from build123d import *

# Parameters (mm, degrees)
F1_DEPTH = 2
F0_R     = 1
F2_DEPTH = 1.2
F3_DEPTH = 5


with BuildPart() as f1:
    # F0 (on Front) → F1 (new body)
    with BuildSketch(Plane.XZ):
        with BuildLine():
            Line((-7.5, -4.5), (7.5, -4.5))
            ThreePointArc((7.5, -4.5), (8.914214, -3.914214), (9.5, -2.5))
            Line((9.5, -2.5), (9.5, 2.5))
            ThreePointArc((9.5, 2.5), (8.914214, 3.914214), (7.5, 4.5))
            Line((7.5, 4.5), (-7.5, 4.5))
            ThreePointArc((-7.5, 4.5), (-8.914214, 3.914214), (-9.5, 2.5))
            Line((-9.5, 2.5), (-9.5, -2.5))
            ThreePointArc((-9.5, -2.5), (-8.914214, -3.914214), (-7.5, -4.5))
        make_face()
        with BuildLine():
            ThreePointArc((8, -1), (7.414214, -2.414214), (6, -3))
            Line((6, -3), (-6, -3))
            ThreePointArc((-6, -3), (-7.414214, -2.414214), (-8, -1))
            Line((-8, -1), (-8, 1))
            ThreePointArc((-8, 1), (-7.414214, 2.414214), (-6, 3))
            Line((-6, 3), (6, 3))
            ThreePointArc((6, 3), (7.414214, 2.414214), (8, 1))
            Line((8, 1), (8, -1))
        make_face(mode=Mode.SUBTRACT)
    extrude(amount=F1_DEPTH)

    # F0 (on Front) → F2 (join)
    with BuildSketch(Plane.XZ):
        with BuildLine():
            Line((-6, -3), (6, -3))
            ThreePointArc((6, -3), (7.414214, -2.414214), (8, -1))
            Line((8, -1), (8, 1))
            ThreePointArc((8, 1), (7.414214, 2.414214), (6, 3))
            Line((6, 3), (-6, 3))
            ThreePointArc((-6, 3), (-7.414214, 2.414214), (-8, 1))
            Line((-8, 1), (-8, -1))
            ThreePointArc((-8, -1), (-7.414214, -2.414214), (-6, -3))
        make_face()
        Circle(F0_R, mode=Mode.SUBTRACT)
    extrude(amount=F2_DEPTH)

    # F0 (on Front) → F3 (join)
    with BuildSketch(Plane.XZ):
        Circle(F0_R)
    extrude(amount=F3_DEPTH)


solid = f1.part
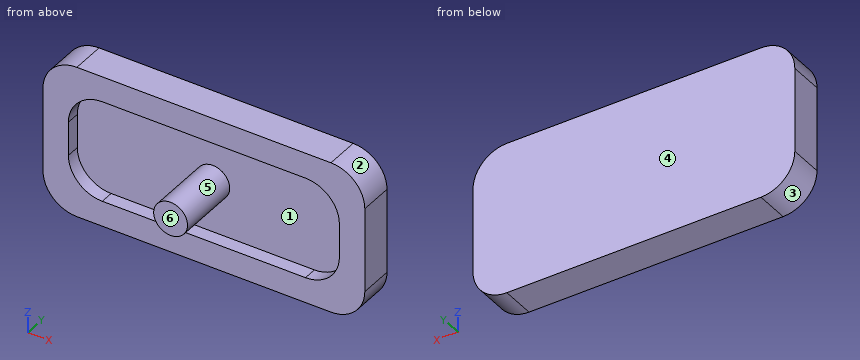
The listing builds one solid part. Answer for the finished solid, in the listing's coordinates (mm). Face numbers are marked on the shaded views. A direction names the side the tool comes from. Give positions to 0.01 mm unless a question says otherwise; leave off trailing zeros. Order: outer loops, then holes, each group sorted by start corner. A loop starts at its lowest first (then second) coordinate and runs counter-clockwise, first axis right, second up. Notation, with made-up numbers: (77.5, 20.5) - (83.5, 20.5) arc R14 ccw to (83.5, 33.5) - close; hole circle Ø7 at (-40, 56.5). An arc over 180 degrees is marked (long way). Use one line per item in the form item = value.
1) The mould has two halves that part along Z. Classify the marked faces 1, 2, 3 and 4: released by +Z, released by -Z, zero draft, split by the parting line, or undercut.
Verdict:
face_1 = undercut
face_2 = released by +Z
face_3 = released by -Z
face_4 = zero draft
2) For the marked faces 5 and 6, determine the directions among +Z, -Z, +X, -X, +Y, -Y from which every point of the face is accessible in a straight line to the end or side of a thin tool.
Verdict:
face_5 = -Y
face_6 = +Z, -Z, +X, -X, -Y
3) Find section B-B on z = 0. Determine the outline of the cut face in (x, y).
Verdict:
outline = (-9.5, -2) - (-8, -2) - (-8, -1.2) - (-1, -1.2) - (-1, -5) - (1, -5) - (1, -1.2) - (8, -1.2) - (8, -2) - (9.5, -2) - (9.5, 0) - (-9.5, 0) - close
4) Find section C-C on y = -4.6. Determine the outline of the cut face in (x, z).
Verdict:
outline = circle Ø2 at (0, 0)
5) Find section A-A on x = 0. Determine the outline of the cut face in (y, z), and give its area (3 significant figures).
Verdict:
outline = (-5, -1) - (-1.2, -1) - (-1.2, -3) - (-2, -3) - (-2, -4.5) - (0, -4.5) - (0, 4.5) - (-2, 4.5) - (-2, 3) - (-1.2, 3) - (-1.2, 1) - (-5, 1) - close
area = 20.8 mm^2
6) Find section D-D on x = -4.25. Determine the outline of the cut face in (y, z).
Verdict:
outline = (-2, -4.5) - (0, -4.5) - (0, 4.5) - (-2, 4.5) - (-2, 3) - (-1.2, 3) - (-1.2, -3) - (-2, -3) - close
7) Each of these flat-tipped pins is pushed along its axis until it touches: pin 1 (1.5 mm diameter, centred on x = 1, z = 1.5, fed in from -Y); pin 2 (1 mm diameter, centred on y = -4, z = 2.5, fed in from +X). Where does it stop, or does it pass through?
Verdict:
pin_1 = -1.2
pin_2 = through
8) Consider probe 1 along Z at (x, y) = (-2.5, -1.25); probe 2 along Y at (x, z) = (-2.75, -0.25); probe 3 along Y at (x, z) = (-8.5, 3.75). Determine where each line is inside the solid, lowest interval first. Write a range as [from, to].
Verdict:
probe_1 = [-4.5, -3], [3, 4.5]
probe_2 = [-1.2, 0]
probe_3 = [-2, 0]
